Geometry check sheet. Reference: drawing and pictorial views, mm from the part's lowest x, y, z. A direction names the side the tool comes from. Round coordinates to 2 decimals unless told otherwise and drop trailing zeros. Order: outer loops, then holes, each group sorted by start corner. A loop starts at its lowest first (then second) coordinate and runs counter-clockwise, first axis right, second up.
(1) Depth check by flat-ended pin: pin 1 (2 mm diameter, centred on y = 12.5, z = 1, fed in from +X). Enter the tip coordinate at first touch or a pass-through.
(2) Thickness scan on probe 1 along Y at (x, z) = (28.5, 1.95); probe 2 along X at (y, z) = (21.5, 1.6). Record the ranges inside material, lowest first.
(3) Sectioned sample at A-A, the plane y = 17.5. Enter the section's corners in (x, z), and give its area (3 significant figures).
(4) Sectioned sample at B-B, the plane z = 1.45. Enter the section's corners in (x, y).
(5) Sectioned sample at C-C, the plane x = 28.5. Enter the section's corners in (y, z).
(6) Tool access check on the marked faces 1 and 2. Record the directions out of +Z, -Z, +X, -X, +Y, -Y that give a thin tool (end or side, any length) a straight path to the whole face; none if there is none.
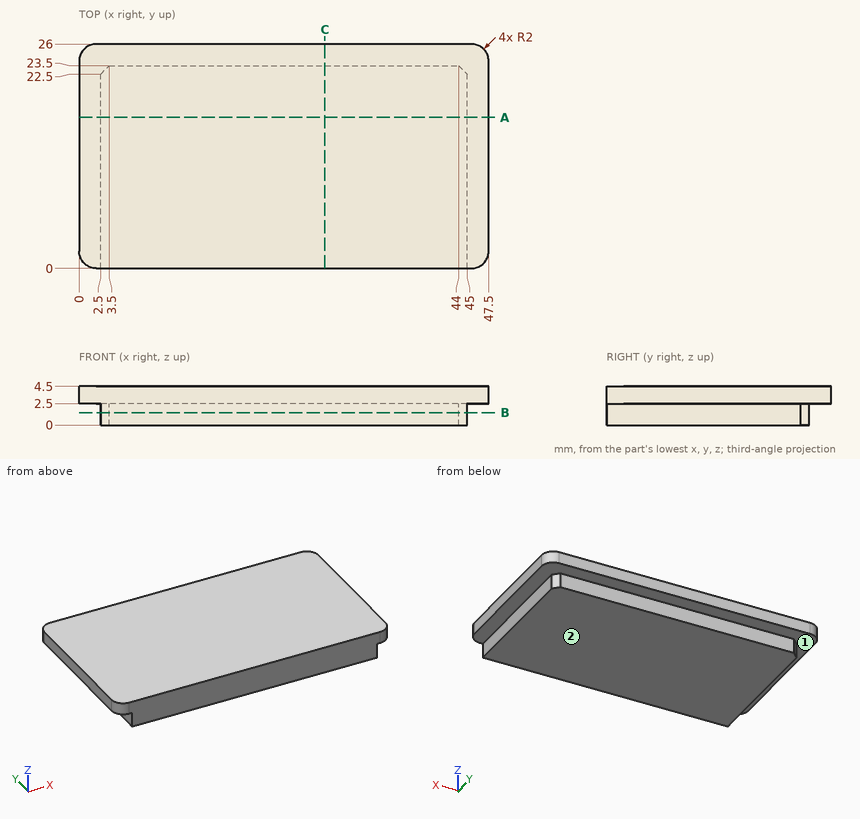
Derived:
1. pin 1: stops at x = 45
2. probe 1: y = 0 to 23.5
2. probe 2: x = 2.5 to 45
3. outline: (0, 2.5) - (2.5, 2.5) - (2.5, 0) - (45, 0) - (45, 2.5) - (47.5, 2.5) - (47.5, 4.5) - (0, 4.5) - close
3. area: 201 mm2
4. outline: (2.5, 0) - (45, 0) - (45, 22.5) - (44, 23.5) - (3.5, 23.5) - (2.5, 22.5) - close
5. outline: (0, 0) - (23.5, 0) - (23.5, 2.5) - (26, 2.5) - (26, 4.5) - (0, 4.5) - close
6. face 1: -Z, +Y
6. face 2: -Z, +X, -X, +Y, -Y
